Geometry check sheet. Reference: the model listing, model coordinates, mm. A direction names the side the tool comes from. Round coordinates to 2 decimals unless told otherwise and drop trailing zeros. Loops run counter-clockwise (first coordinate to the right, second up) from the corner with the lowest first, then second, coordinate; pieces in that order, holes last. Notation, with made-up numbers: (-11.5, -36.5) -> (-3.5, -36.5) arc R22 ccw to (-3.5, -18.5) -> close; hole circle Ø10 at (-36, 42.5). An arc over 180 degrees is marked (long way). Use one line per item in the form item = value.
from build123d import *

# Parameters (mm, degrees)
SKETCH_1_R               = 10
EXTRUDE_1_DEPTH          = 250
SKETCH_6_R               = 16
EXTRUDE_2_DEPTH          = 18
CUT_EXTRUDE_START        = 30
SKETCH_2_R               = 6
CUT_EXTRUDE_1_DEPTH      = 260
M14X1_5_1_D              = 12.5
M14X1_5_1_DEPTH          = 35
M14X1_5_1_TIP            = 3.755378869
CHAMFER_1_SIZE           = 1.5
SKETCH_8_R               = 8
CUT_EXTRUDE_2_DEPTH      = 15.5
HOLE_WIZARD_M3_1_D       = 2.5
HOLE_WIZARD_M3_1_DEPTH   = 25
HOLE_WIZARD_M3_1_TIP     = 0.751075774
CUT_EXTRUDE_1_2_DEPTH    = 252.021911394
PATTERN_CIRCULAR_1_COUNT = 4
CHAMFER_2_SIZE           = 0.8


with BuildPart() as part:
    # 草图1 → 凸台-拉伸1 (new body)
    with BuildSketch(Plane(origin=(0, 0, 0), x_dir=(1, 0, 0), z_dir=(0, 1, 0))):
        with Locations(Location((0, 0, 0), (0, 0, 270))):
            Circle(SKETCH_1_R)
    extrude(amount=EXTRUDE_1_DEPTH)

    # 草图6 → 凸台-拉伸2 (add)
    with BuildSketch(Plane.XZ):
        with Locations(Location((0, 0, 0), (0, 0, 270))):
            Circle(SKETCH_6_R)
    extrude(amount=-EXTRUDE_2_DEPTH)

    # 草图2 → Cut-Extrude 1 (cut)
    with BuildSketch(Plane.XZ.offset(-250).offset(CUT_EXTRUDE_START)):
        with Locations(Location((0, 0, 0), (0, 0, 90))):
            Circle(SKETCH_2_R)
    extrude(amount=CUT_EXTRUDE_1_DEPTH, mode=Mode.SUBTRACT)

    # M14x1.5 螺纹孔1
    with Locations(Plane(origin=(0, 250, 0), x_dir=(1, 0, 0), z_dir=(0, 1, 0))):
        with Locations((0, 0)):
            Hole(M14X1_5_1_D / 2, depth=M14X1_5_1_DEPTH)
            with Locations((0, 0, -(M14X1_5_1_DEPTH + M14X1_5_1_TIP / 2))):  # 118° drill point
                Cone(0, M14X1_5_1_D / 2, M14X1_5_1_TIP, mode=Mode.SUBTRACT)

    # 倒角1
    chamfer_1_edges = [part.edges().sort_by_distance(p)[0] for p in [
        (6.25, 250, 0),
    ]]
    chamfer(chamfer_1_edges, length=CHAMFER_1_SIZE)

    # 草图8 → 切除-拉伸2 (cut)
    with BuildSketch(Plane.XZ):
        with Locations(Location((0, 0, 0), (0, 0, 270))):
            Circle(SKETCH_8_R)
    extrude(amount=-CUT_EXTRUDE_2_DEPTH, mode=Mode.SUBTRACT)

    # M3 螺纹孔1
    with Locations(Plane(origin=(0, 0, 0), x_dir=(-1, 0, 0), z_dir=(0, -1, 0))):
        with Locations((0, 12), (12, 0), (0, -12), (-12, 0)):
            Hole(HOLE_WIZARD_M3_1_D / 2, depth=HOLE_WIZARD_M3_1_DEPTH)
            with Locations((0, 0, -(HOLE_WIZARD_M3_1_DEPTH + HOLE_WIZARD_M3_1_TIP / 2))):  # 118° drill point
                Cone(0, HOLE_WIZARD_M3_1_D / 2, HOLE_WIZARD_M3_1_TIP, mode=Mode.SUBTRACT)

    # 草图13 → Cut-Extrude 1 2 (cut, symmetric)
    with BuildSketch(Plane.XZ):
        Polygon((-8.62670273, 10.88944443), (-10.182337649, 12.445079349), (-12.445079349, 10.182337649), (-10.88944443, 8.62670273), align=None)
    cut_extrude_1_2 = extrude(amount=CUT_EXTRUDE_1_2_DEPTH, both=True, mode=Mode.SUBTRACT)

    # 阵列(圆周)1: Cut-Extrude 1 2 ×4 about axis
    pattern_circular_1_axis = Axis((0, 0, 0), (0, 1, 0))
    for i in range(1, PATTERN_CIRCULAR_1_COUNT):
        add(cut_extrude_1_2.rotate(pattern_circular_1_axis, i * 360 / PATTERN_CIRCULAR_1_COUNT), mode=Mode.SUBTRACT)

    # 倒角2
    chamfer_2_edges = [part.edges().sort_by_distance(p)[0] for p in [
        (0, 250, -10),
    ]]
    chamfer(chamfer_2_edges, length=CHAMFER_2_SIZE)


solid = part.part
1. Section check A-A (y = 29.5). Record the boundary of the cut face in (x, z).
Return value:
outline = circle Ø20 at (0, 0); hole circle Ø12 at (0, 0)
2. Tool access check on faces 1 (the flat face through (3.8, 0, 7.3)), 2 (the cylindrical face through (-9.76, 131.98, -2.17)), 3 (the flat face through (6, 15.5, 2)). Record the directions out of +Z, -Z, +X, -X, +Y, -Y that give a thin tool (end or side, any length) a straight path to the whole face; none if there is none.
Return value:
face_1 = +Z, -Z, +X, -X, -Y
face_2 = +Y
face_3 = -Y
3. Mould release check, pull along Z, two halves, no side actions. Record for faces 4 (the flat face through (-7, 250, -4)), 5 (the cylindrical face through (16, 9, 0)), 6 (the cylindrical face through (-5.96, 231.52, -1.88)): released by +Z, released by -Z, zero draft, split by the parting line, or undercut.
Return value:
face_4 = zero draft
face_5 = split by the parting line
face_6 = undercut
4. Gauge pin test, flat ends, axial feed: pin 1 (10 mm diameter, centred on x = -3, y = 45, fed in from +Z); pin 2 (1 mm diameter, centred on x = 8, y = 139.5, fed in from -Z); pin 3 (10 mm diameter, centred on y = 41, z = -0.5, fed in from +X). Record the tip position at first contact, or that the pin passes through.
Return value:
pin_1 = 10
pin_2 = -6.61
pin_3 = 10
5. Material ranges on line 1 along X through (y, z) = (167, 0); line 2 along Y through (x, z) = (3.5, 14.5); line 3 along X through (y, z) = (62, 3), recorded low to high.
Return value:
line_1 = -10 to -6, 6 to 10
line_2 = 0 to 18
line_3 = -9.54 to -5.2, 5.2 to 9.54
